```python
from build123d import *

# Parameters (mm, degrees)
F0_R      = 32.5501
F2_R      = 30.9626
F7_R      = 24.6126
F7_R_2    = 23.0251
F8_DEPTH  = 1.5875
F13_R     = 10.3251
F14_DEPTH = 11.0998
F17_D     = 12.7
F18_R     = 2.5527
F19_DEPTH = 25.4
F21_R     = 5.1562
F22_DEPTH = 25.4


with BuildPart() as f3:
    # F0 (on Top) → F3 section 0
    with BuildSketch(Plane.XY):
        Circle(F0_R)
    # F2 (on offset) → F3 section 1
    with BuildSketch(Plane.XY.offset(20.6502)):
        Circle(F2_R)
    loft()


with BuildPart() as f5:
    # F4 (on Front) → F5 (revolve)
    with BuildSketch(Plane.XZ):
        Polygon((30.9626, 20.6502), (0, 20.6502), (0, 19.0627), (24.595485268, 19.0627), align=None)
    revolve(axis=Axis((0, 0, 0), (0, 0, 1)))


with BuildPart() as f3_1:
    add(f3.part)

    # F6: cut F5
    add(f5.part, mode=Mode.SUBTRACT)


with BuildPart() as f8:
    # F7 (on face) → F8 (new body, symmetric)
    with BuildSketch(Plane.XY.offset(19.0627)):
        Circle(F7_R)
        Circle(F7_R_2, mode=Mode.SUBTRACT)
    extrude(amount=F8_DEPTH, both=True)


with BuildPart() as f3_2:
    add(f3_1.part)

    # F9: cut F8
    add(f8.part, mode=Mode.SUBTRACT)


with BuildPart() as f11:
    # F10 (on Front) → F11 (revolve)
    with BuildSketch(Plane.XZ):
        Polygon((23.0251, 19.0627), (0, 19.0627), (0, 15.8877), (15.1666992404, 15.8877), align=None)
    revolve(axis=Axis((0, 0, 0), (0, 0, 1)))


with BuildPart() as f3_3:
    add(f3_2.part)

    # F12: cut F11
    add(f11.part, mode=Mode.SUBTRACT)


with BuildPart() as f14:
    # F13 (on face) → F14 (new body, symmetric)
    with BuildSketch(Plane.XY.offset(15.8877)):
        Circle(F13_R)
    extrude(amount=F14_DEPTH, both=True)


with BuildPart() as f3_4:
    add(f3_3.part)

    # F15: cut F14
    add(f14.part, mode=Mode.SUBTRACT)

    # F17 (through all)
    with Locations(Plane.XY.offset(4.7879)):
        with Locations((0, 0)):
            Hole(F17_D / 2)


with BuildPart() as f19:
    # F18 (on offset) → F19 (new body, symmetric)
    with BuildSketch(Plane.XY.offset(20.6502)):
        with Locations((17.4752, 0)):
            Circle(F18_R)
    extrude(amount=F19_DEPTH, both=True)


with BuildPart() as f3_5:
    add(f3_4.part)

    # F20: cut F19
    add(f19.part, mode=Mode.SUBTRACT)


with BuildPart() as f22:
    # F21 (on Top) → F22 (new body)
    with BuildSketch(Plane.XY):
        with Locations((17.4752, 0)):
            Circle(F21_R)
    extrude(amount=F22_DEPTH)


with BuildPart() as f22_1:
    # F23: moved
    add(f22.part.moved(Location((0, 0, 4.7752))))


with BuildPart() as f3_6:
    add(f3_5.part)

    # F24: cut F22
    add(f22_1.part, mode=Mode.SUBTRACT)


solid = f3_6.part
```
CAD build for the part. Positions are in the model's coordinates, mm. A direction names the side the tool comes from. Coordinates: 2 decimals unless noted, no trailing zeros. Write each loop counter-clockwise with the first axis right and the second up, starting at its lowest first coordinate (ties: lowest second). Pieces come first, ordered by that corner, then holes. Notation, with made-up numbers: (57, -0.5) -> (62, -0.5) arc R14 ccw to (62, 6.5) -> close; hole circle Ø8 at (70.5, -9.75). An arc over 180 degrees is marked (long way). Return JSON: item names as keys, results as strings. Group by question number.
Q1. Flat gauge pins, fed straight in: pin 1 (1 mm diameter, centred on y = 6, z = 14, fed in from +X); pin 2 (16.5 mm diameter, centred on x = 0, y = 0, fed in from +Z); pin 3 (15 mm diameter, centred on x = -7, y = 12, fed in from +Z). Where does each tip first touch, or does it go through?
Q2. Cut at A-A, the plane x = 0. Give the cut face in (y, z), then the cut area to 3 significant figures.
Q3. Cut at B-B, the plane y = 0. State how many separate pieces and enclosed holes the cut face has, then the cut area to 3 significant figures.
Q4. Which spindle directions (+Z, -Z, +X, -X, +Y, -Y) get a long thin tool onto all of the face, cutting with end or side? Do faces 4 (the face through (14.5, -18.1, 17.475)), 5 (the face through (14.925, 0.112, 2.421)). Say none if no direction does.
Q5. Cut at C-C, the plane z = 12.5. Give the cut face in (x, y), then the cut area to 3 significant figures.
Q6. Pull direction X, two halves, no side cores. Call faces 1 (the face through (30.111, 9.482, 12.764)), 2 (the face through (0, -7, 0)), 3 (the face through (20, -2, 4.775)): released by +X, released by -X, zero draft, split by the parting line, or undercut.
Q7. Drill centre lines: line 1 (X direction, y = 0.5, z = 7.5); line 2 (Z direction, x = -21, y = 11.5); line 3 (Y direction, x = 0, z = 1.45). Where is each one in solid material? Low to high.
Q8. Cut at D-D, the plane z = 2.25. Give the cut face in (x, y), then the cut area to 3 significant figures.
Returned:
{
 "1": {"pin 1": "stops at x = 31", "pin 2": "stops at z = 4.79", "pin 3": "stops at z = 18.4"},
 "2": {"outline": "(-32.55, 0) -> (-6.35, 0) -> (-6.35, 4.79) -> (-10.33, 4.79) -> (-10.33, 15.89) -> (-15.17, 15.89) -> (-23.03, 19.06) -> (-23.03, 17.48) -> (-24.61, 17.48) -> (-24.61, 19.07) -> (-30.96, 20.65) -> close; (6.35, 0) -> (32.55, 0) -> (30.96, 20.65) -> (24.61, 19.07) -> (24.61, 17.48) -> (23.03, 17.48) -> (23.03, 19.06) -> (15.17, 15.89) -> (10.33, 15.89) -> (10.33, 4.79) -> (6.35, 4.79) -> close", "area": "807 mm2"},
 "3": {"separate pieces": "3", "enclosed holes": "0", "area": "657 mm2"},
 "4": {"face 4": "+Z", "face 5": "+Z, -Z"},
 "5": {"outline": "circle Ø63.18 at (0, 0); hole circle Ø20.65 at (0, 0); hole circle Ø10.31 at (17.48, 0)", "area": "2,720 mm2"},
 "6": {"face 1": "split by the parting line", "face 2": "zero draft", "face 3": "undercut"},
 "7": {"line 1": "x = -31.97 to -10.31, 10.31 to 12.34, 22.61 to 31.97", "line 2": "z = 0 to 17.48", "line 3": "y = -32.44 to -6.35, 6.35 to 32.44"},
 "8": {"outline": "circle Ø64.75 at (0, 0); hole circle Ø12.7 at (0, 0); hole circle Ø5.11 at (17.48, 0)", "area": "3,150 mm2"}
}
